Could you check a few things on this model? Use its own coordinates, in mm. A direction names the side the tool comes from. Give positions to 0.01 mm unless a question says otherwise; leave off trailing zeros. Write each loop counter-clockwise with the first axis right and the second up, starting at its lowest first coordinate (ties: lowest second). Pieces come first, ordered by that corner, then holes. Notation, with made-up numbers: (70.25, 12.25) - (78.25, 12.25) arc R25 ccw to (78.25, 42.25) - close; hole circle Ø7 at (-32.75, -20.75). An arc over 180 degrees is marked (long way). Answer in a Markdown table with one row per item.
from build123d import *

# Parameters (mm, degrees)
CYLINDER975_R          = 1.25
CYLINDER975_DEPTH      = 4
CYLINDER975_ROLL_ANGLE = 90
CYLINDER979_R          = 1.25
CYLINDER979_DEPTH      = 7
CYLINDER977_R          = 2.6
CYLINDER977_DEPTH      = 11
CYLINDER977_ROLL_ANGLE = 90
CYLINDER981_R          = 1.25
CYLINDER981_DEPTH      = 4
CYLINDER981_ROLL_ANGLE = 90
CYLINDER976_R          = 5.6
CYLINDER976_DEPTH      = 4
CYLINDER976_ROLL_ANGLE = 90
CYLINDER978_R          = 8
CYLINDER978_DEPTH      = 6
CYLINDER978_ROLL_ANGLE = 90
BOX566_W               = 6
BOX566_H               = 4
BOX566_DEPTH           = 16.5
CYLINDER973_R          = 7
CYLINDER973_DEPTH      = 6
CYLINDER973_ROLL_ANGLE = 90
BOX565_W               = 6
BOX565_H               = 4
BOX565_DEPTH           = 22
CYLINDER980_R          = 4
CYLINDER980_DEPTH      = 4
CYLINDER980_ROLL_ANGLE = 90
CYLINDER974_R          = 4
CYLINDER974_DEPTH      = 4
CYLINDER974_ROLL_ANGLE = 90
CHAMFER106_SIZE        = 0.999


with BuildPart() as cylinder1154:
    # Cylinder975 → Cylinder975 (new body)
    with BuildSketch(Plane.XY):
        Circle(CYLINDER975_R)
    extrude(amount=CYLINDER975_DEPTH)


with BuildPart() as cylinder1154_1:
    # Cylinder975 roll: moved
    add(cylinder1154.part.rotate(Axis((0, 0, 0), (1, 0, 0)), CYLINDER975_ROLL_ANGLE))


with BuildPart() as cylinder1154_2:
    # Cylinder975 placement: moved
    add(cylinder1154_1.part.moved(Location((37, 32.75, -33))))


with BuildPart() as cylinder1158:
    # Cylinder979 → Cylinder979 (new body)
    with BuildSketch(Plane(origin=(37, 37.75, -8), x_dir=(1, 0, 0), z_dir=(0, 0, 1))):
        Circle(CYLINDER979_R)
    extrude(amount=CYLINDER979_DEPTH)


with BuildPart() as cylinder1156:
    # Cylinder977 → Cylinder977 (new body)
    with BuildSketch(Plane.XY):
        Circle(CYLINDER977_R)
    extrude(amount=CYLINDER977_DEPTH)


with BuildPart() as cylinder1156_1:
    # Cylinder977 roll: moved
    add(cylinder1156.part.rotate(Axis((0, 0, 0), (1, 0, 0)), CYLINDER977_ROLL_ANGLE))


with BuildPart() as cylinder1156_2:
    # Cylinder977 placement: moved
    add(cylinder1156_1.part.moved(Location((37, 39.75, -11))))


with BuildPart() as cylinder1160:
    # Cylinder981 → Cylinder981 (new body)
    with BuildSketch(Plane.XY):
        Circle(CYLINDER981_R)
    extrude(amount=CYLINDER981_DEPTH)


with BuildPart() as cylinder1160_1:
    # Cylinder981 roll: moved
    add(cylinder1160.part.rotate(Axis((0, 0, 0), (1, 0, 0)), CYLINDER981_ROLL_ANGLE))


with BuildPart() as cylinder1160_2:
    # Cylinder981 placement: moved
    add(cylinder1160_1.part.moved(Location((37, 32.75, 5.5))))


with BuildPart() as fusion612:
    # Cylinder976 → Cylinder976 (new body)
    with BuildSketch(Plane.XY):
        Circle(CYLINDER976_R)
    extrude(amount=CYLINDER976_DEPTH)


with BuildPart() as fusion612_1:
    # Cylinder976 roll: moved
    add(fusion612.part.rotate(Axis((0, 0, 0), (1, 0, 0)), CYLINDER976_ROLL_ANGLE))


with BuildPart() as fusion612_2:
    # Cylinder976 placement: moved
    add(fusion612_1.part.moved(Location((37, 39.75, -11))))

    # Fusion612: union Cylinder1154, Cylinder1158, Cylinder1156, Cylinder1160
    add(cylinder1154_2.part)
    add(cylinder1158.part)
    add(cylinder1156_2.part)
    add(cylinder1160_2.part)


with BuildPart() as cylinder1157:
    # Cylinder978 → Cylinder978 (new body)
    with BuildSketch(Plane.XY):
        Circle(CYLINDER978_R)
    extrude(amount=CYLINDER978_DEPTH)


with BuildPart() as cylinder1157_1:
    # Cylinder978 roll: moved
    add(cylinder1157.part.rotate(Axis((0, 0, 0), (1, 0, 0)), CYLINDER978_ROLL_ANGLE))


with BuildPart() as cylinder1157_2:
    # Cylinder978 placement: moved
    add(cylinder1157_1.part.moved(Location((37, 39.75, -11))))


with BuildPart() as cube757:
    # Box566 → Box566 (new body)
    with BuildSketch(Plane(origin=(34, 33.75, -11), x_dir=(1, 0, 0), z_dir=(0, 0, 1))):
        with Locations((3, 2)):
            Rectangle(BOX566_W, BOX566_H)
    extrude(amount=BOX566_DEPTH)


with BuildPart() as cylinder1152:
    # Cylinder973 → Cylinder973 (new body)
    with BuildSketch(Plane.XY):
        Circle(CYLINDER973_R)
    extrude(amount=CYLINDER973_DEPTH)


with BuildPart() as cylinder1152_1:
    # Cylinder973 roll: moved
    add(cylinder1152.part.rotate(Axis((0, 0, 0), (1, 0, 0)), CYLINDER973_ROLL_ANGLE))


with BuildPart() as cylinder1152_2:
    # Cylinder973 placement: moved
    add(cylinder1152_1.part.moved(Location((37, 39.75, -11))))


with BuildPart() as cube756:
    # Box565 → Box565 (new body)
    with BuildSketch(Plane(origin=(34, 33.75, -33), x_dir=(1, 0, 0), z_dir=(0, 0, 1))):
        with Locations((3, 2)):
            Rectangle(BOX565_W, BOX565_H)
    extrude(amount=BOX565_DEPTH)


with BuildPart() as cylinder1159:
    # Cylinder980 → Cylinder980 (new body)
    with BuildSketch(Plane.XY):
        Circle(CYLINDER980_R)
    extrude(amount=CYLINDER980_DEPTH)


with BuildPart() as cylinder1159_1:
    # Cylinder980 roll: moved
    add(cylinder1159.part.rotate(Axis((0, 0, 0), (1, 0, 0)), CYLINDER980_ROLL_ANGLE))


with BuildPart() as cylinder1159_2:
    # Cylinder980 placement: moved
    add(cylinder1159_1.part.moved(Location((37, 37.75, 5.5))))


with BuildPart() as front_axle_steering_arm_with_rear_link:
    # Cylinder974 → Cylinder974 (new body)
    with BuildSketch(Plane.XY):
        Circle(CYLINDER974_R)
    extrude(amount=CYLINDER974_DEPTH)


with BuildPart() as front_axle_steering_arm_with_rear_link_1:
    # Cylinder974 roll: moved
    add(front_axle_steering_arm_with_rear_link.part.rotate(Axis((0, 0, 0), (1, 0, 0)), CYLINDER974_ROLL_ANGLE))


with BuildPart() as front_axle_steering_arm_with_rear_link_2:
    # Cylinder974 placement: moved
    add(front_axle_steering_arm_with_rear_link_1.part.moved(Location((37, 37.75, -33))))

    # Fusion611: union Cube757, Cylinder1152, Cube756, Cylinder1159
    add(cube757.part)
    add(cylinder1152_2.part)
    add(cube756.part)
    add(cylinder1159_2.part)


with BuildPart() as front_axle_steering_arm_with_rear_link_3:
    # Fusion611 placement: moved
    add(front_axle_steering_arm_with_rear_link_2.part.moved(Location((0, -5, 0))))

    # Fusion613: union Cylinder1157
    add(cylinder1157_2.part)

    # Cut702: cut Fusion612
    add(fusion612_2.part, mode=Mode.SUBTRACT)

    # Chamfer106
    chamfer106_edges = [front_axle_steering_arm_with_rear_link_3.edges().sort_by_distance(p)[0] for p in [
        (30, 33.75, -11),
    ]]
    chamfer(chamfer106_edges, length=CHAMFER106_SIZE)


solid = front_axle_steering_arm_with_rear_link_3.part
1) Imagine slicing it at A-A (x = 37). State how many separate pieces and enclosed holes the cut face has, then the cut area to 3 significant figures.
Check values:
| item | result |
|---|---|
| separate pieces | 5 |
| enclosed holes | 0 |
| area | 190 mm2 |
2) Will these pins go through, and if not, where does the flat tip stop? P1, Ø4.5, axis at y = 31, z = 0.5, coming from the -X side; P2, Ø4, axis at x = 37, z = -33, coming from the +Y side; P3, Ø8.5, axis at x = 37, z = -11, coming from the +Y side; P4, Ø4, axis at y = 35, z = -26, coming from the -X side (3 decimals).
Check values:
| item | result |
|---|---|
| P1 | stops at x = 34 |
| P2 | stops at y = 32.75 |
| P3 | stops at y = 35.75 |
| P4 | passes through |
3) Imagine slicing it at C-C (y = 31). List the corners of the cut face in (x, z) for me, then the cut area to 3 significant figures.
Check values:
| item | result |
|---|---|
| outline | (34, -30.35) arc R4 ccw (long way) to (40, -30.35) - (40, -17.32) arc R7 ccw to (40, -4.68) - (40, 2.85) arc R4 ccw (long way) to (34, 2.85) - (34, -4.68) arc R7 ccw to (34, -17.32) - close; hole circle Ø5.2 at (37, -11); hole circle Ø2.5 at (37, -33); hole circle Ø2.5 at (37, 5.5) |
| area | 330 mm2 |
4) Imagine slicing it at B-B (z = -33). List the corners of the cut face in (x, y) for me, then the cut area to 3 significant figures.
Check values:
| item | result |
|---|---|
| outline | (33, 28.75) - (35.75, 28.75) - (35.75, 32.75) - (33, 32.75) - close; (38.25, 28.75) - (41, 28.75) - (41, 32.75) - (38.25, 32.75) - close |
| area | 22.0 mm2 |
5) If I drill on line 1 (Z direction, x = 37, y = 31.5); line 2 (Z direction, x = 37, y = 36); line 3 (Z direction, x = 37, y = 38), over which ranges is the centre line in solid material (lowest first)?
Check values:
| item | result |
|---|---|
| line 1 | z = -37 to -34.25, -31.75 to -13.6, -8.4 to 4.25, 6.75 to 9.5 |
| line 2 | z = -19 to -16.6, -5.4 to -3 |
| line 3 | z = -19 to -16.6 |
6) Imagine slicing it at D-D (z = -24). List the corners of the cut face in (x, y) for me, then the cut area to 3 significant figures.
Check values:
| item | result |
|---|---|
| outline | (34, 28.75) - (40, 28.75) - (40, 32.75) - (34, 32.75) - close |
| area | 24.0 mm2 |
7) We'd pull the mould along X, two halves only. Please class faces 1 (the face through (31.55, 39.75, -9.11)), 2 (the face through (38, 35.75, -8)), 3 (the face through (34, 31, -1)): +X half, -X half, draft (parallel to the pull), parting line (faces both ways), or undercut.
Check values:
| item | result |
|---|---|
| face 1 | draft |
| face 2 | undercut |
| face 3 | -X half |
8) On a 3-axis mill with a long thin cutter (end or side, diameter ignored), from which of +Z, -Z, +X, -X, +Y, -Y can I reach the whole of each face in a straight line? I mean faces 4 (the face through (34.937, 32.299, -12.582)), 5 (the face through (38.2, 38.1, -4.3)), 6 (the face through (43.466, 30.779, -13.681)), 7 (the face through (35.27, 36.79, -18.81)). Say none if no direction works.
Check values:
| item | result |
|---|---|
| face 4 | +Y, -Y |
| face 5 | +Z |
| face 6 | -Y |
| face 7 | +Y |
